```python
from build123d import *

# Parameters (mm, degrees)
SKETCH1_W           = 187
SKETCH1_H           = 50
BOSS_EXTRUDE1_DEPTH = 5
SKETCH2_R           = 3
CUT_EXTRUDE1_DEPTH  = 5
SKETCH3_R           = 2.5
CUT_EXTRUDE2_DEPTH  = 5
SKETCH4_R           = 2.5
CUT_EXTRUDE3_DEPTH  = 25
SKETCH5_R           = 2.5
CUT_EXTRUDE4_DEPTH  = 25


with BuildPart() as part:
    # Sketch1 → Boss-Extrude1 (new body)
    with BuildSketch(Plane(origin=(0, 0, 0), x_dir=(1, 0, 0), z_dir=(0, 1, 0))):
        with Locations((93.5, 25)):
            Rectangle(SKETCH1_W, SKETCH1_H)
    extrude(amount=BOSS_EXTRUDE1_DEPTH)

    # Sketch2 → Cut-Extrude1 (cut)
    with BuildSketch(Plane(origin=(0, 5, 0), x_dir=(1, 0, 0), z_dir=(0, 1, 0))):
        with Locations(Location((65, 25, 0), (0, 0, 270))):
            Circle(SKETCH2_R)
        with Locations(Location((122, 25, 0), (0, 0, 270))):
            Circle(SKETCH2_R)
    extrude(amount=-CUT_EXTRUDE1_DEPTH, mode=Mode.SUBTRACT)

    # Sketch3 → Cut-Extrude2 (cut)
    with BuildSketch(Plane(origin=(0, 5, 0), x_dir=(1, 0, 0), z_dir=(0, 1, 0))):
        with Locations(Location((144.5, 40.5, 0), (0, 0, 270))):
            Circle(SKETCH3_R)
        with Locations(Location((144.5, 9.5, 0), (0, 0, 270))):
            Circle(SKETCH3_R)
        with Locations(Location((179.5, 9.5, 0), (0, 0, 270))):
            Circle(SKETCH3_R)
        with Locations(Location((179.5, 40.5, 0), (0, 0, 270))):
            Circle(SKETCH3_R)
    extrude(amount=-CUT_EXTRUDE2_DEPTH, mode=Mode.SUBTRACT)

    # Sketch4 → Cut-Extrude3 (cut)
    with BuildSketch(Plane(origin=(0, 5, 0), x_dir=(1, 0, 0), z_dir=(0, 1, 0))):
        with Locations(Location((7.5, 40.5, 0), (0, 0, 270))):
            Circle(SKETCH4_R)
    extrude(amount=-CUT_EXTRUDE3_DEPTH, mode=Mode.SUBTRACT)

    # Sketch5 → Cut-Extrude4 (cut)
    with BuildSketch(Plane(origin=(0, 5, 0), x_dir=(1, 0, 0), z_dir=(0, 1, 0))):
        with Locations(Location((42.5, 9.5, 0), (0, 0, 270))):
            Circle(SKETCH5_R)
        with Locations(Location((7.5, 9.5, 0), (0, 0, 270))):
            Circle(SKETCH5_R)
        with Locations(Location((42.5, 40.5, 0), (0, 0, 270))):
            Circle(SKETCH5_R)
    extrude(amount=-CUT_EXTRUDE4_DEPTH, mode=Mode.SUBTRACT)


solid = part.part
```
Geometry: final body of the model. Coordinates: model frame, mm. Round coordinates to 2 decimals unless told otherwise and drop trailing zeros. Write each loop counter-clockwise with the first axis right and the second up, starting at its lowest first coordinate (ties: lowest second). Pieces come first, ordered by that corner, then holes.
Item 1: Section query D-D (z = -9.5). Return loops of the section in (x, y).
Item 2: Material intervals for L1, parallel to X at y = 1.3, z = -9.5; L2, parallel to Z at x = 144.5, y = 3.1; L3, parallel to X at y = 3.55, z = -25, sorted ascending.
Item 3: Section query C-C (y = 2.2). Give the number of separate pieces and of enclosed holes in the cut face, plus the area to 3 significant figures.
Item 4: Section query B-B (x = 179.5). Return loops of the section in (y, z), plus the area to 3 significant figures.
Item 5: Section query A-A (z = -25). Return loops of the section in (x, y).
Item 6: Mould query, pull axis X, two halves, no side actions, for faces 1 (the face through (92, 0, -25)), 2 (the face through (146.61, 2.54, -39.16)), 3 (the face through (0, 2, -25)). Classes: +X half, -X half, draft (parallel to the pull), parting line (faces both ways), or undercut.
Completed:
1. outline: (0, 0) - (5, 0) - (5, 5) - (0, 5) - close; (10, 0) - (40, 0) - (40, 5) - (10, 5) - close; (45, 0) - (142, 0) - (142, 5) - (45, 5) - close; (147, 0) - (177, 0) - (177, 5) - (147, 5) - close; (182, 0) - (187, 0) - (187, 5) - (182, 5) - close
2. L1: x = 0 to 5, 10 to 40, 45 to 142, 147 to 177, 182 to 187
2. L2: z = -50 to -43, -38 to -12, -7 to 0
2. L3: x = 0 to 62, 68 to 119, 125 to 187
3. separate pieces: 1
3. enclosed holes: 10
3. area: 9,140 mm2
4. outline: (0, -50) - (5, -50) - (5, -43) - (0, -43) - close; (0, -38) - (5, -38) - (5, -12) - (0, -12) - close; (0, -7) - (5, -7) - (5, 0) - (0, 0) - close
4. area: 200 mm2
5. outline: (0, 0) - (62, 0) - (62, 5) - (0, 5) - close; (68, 0) - (119, 0) - (119, 5) - (68, 5) - close; (125, 0) - (187, 0) - (187, 5) - (125, 5) - close
6. face 1: draft
6. face 2: undercut
6. face 3: -X half
